Work out the finished part from the listing and answer in its coordinate system (mm). Give positions to 0.01 mm unless a question says otherwise; leave off trailing zeros. Loops run counter-clockwise (first coordinate to the right, second up) from the corner with the lowest first, then second, coordinate; pieces in that order, holes last. Notation, with made-up numbers: (45.25, -24) - (90.25, -24) arc R9 ccw to (90.25, -18) - close; hole circle Ø10 at (63, 83). An arc over 180 degrees is marked (long way). One line per item, written item: value.
from build123d import *

# Parameters (mm, degrees)
PAD_DEPTH    = 0.046
SKETCH002_W  = 1.924742
SKETCH002_H  = 2.351108
PAD001_DEPTH = 0.05
SKETCH003_W  = 0.414509
SKETCH003_H  = 1.190033
PAD002_DEPTH = 0.05


with BuildPart() as part:
    # Sketch → Pad (new body)
    with BuildSketch(Plane.XY):
        Polygon((36.346094, 51.80915), (36.392998, 51.701576), (36.392998, 51.109999), (37.742998, 51.109999), (37.742998, 51.259997), (38.392999, 51.259997), (38.392999, 49.31), (35.458194, 49.31), (35.4573, 49.310176), (35.427625, 49.310087), (35.398525, 49.315875), (34.512999, 49.315875), (34.395946, 49.292591), (34.296711, 49.226287), (34.230407, 49.127052), (34.207122, 49.009999), (34.207122, 45.461999), (34.230407, 45.344946), (34.296711, 45.245711), (34.386002, 45.186051), (34.386002, 44.708), (34.642999, 44.708), (34.642999, 44.322444), (34.615783, 44.295228), (34.565999, 44.175042), (34.565999, 44.044954), (34.615783, 43.924769), (34.642999, 43.897553), (34.642999, 38.31), (34.992186, 38.31), (34.992186, 36.056903), (36.893, 36.056903), (36.893, 35.478903), (36.871742, 35.372032), (36.871742, 33.780103), (36.890262, 33.687001), (36.860833, 33.559999), (33.906066, 33.559999), (33.906066, 35.790099), (33.069934, 35.790099), (33.069934, 34.437018), (33.064958, 34.412001), (33.064958, 33.673212), (32.951745, 33.559999), (31.092999, 33.559999), (31.092999, 50.109999), (28.362245, 50.109999), (28.362245, 53.56), (31.439899, 53.56), (31.439899, 51.809147), align=None)
    extrude(amount=PAD_DEPTH)

    # Sketch002 (on Face52 of Pad) → Pad001 (join)
    with BuildSketch(Plane.XY.offset(0.046)):
        with Locations((29.62901, 51.992506)):
            Rectangle(SKETCH002_W, SKETCH002_H)
    extrude(amount=PAD001_DEPTH)

    # Sketch003 (on Face5 of Pad001) → Pad002 (join)
    with BuildSketch(Plane.XY.offset(0.046)):
        with Locations((34.881022, 34.35564)):
            Rectangle(SKETCH003_W, SKETCH003_H)
    extrude(amount=PAD002_DEPTH)


solid = part.part
1. A flat-ended cylindrical pin translates along its axis: pin 1 Ø1.5 at (x, y) = (32.5, 42.5) entering from +Z. Find the tip coordinate at first contact, or state that the pin passes through.
Output:
pin 1: stops at z = 0.05
2. Section C-C (y = 46.75) is taken. Write down the section's boundary in (x, z), and give its area (3 significant figures).
Output:
outline: (31.09, 0) - (34.21, 0) - (34.21, 0.05) - (31.09, 0.05) - close
area: 0.143 mm²
3. Section A-A (x = 29.75) is taken. Write down the section's boundary in (y, z).
Output:
outline: (50.11, 0) - (53.56, 0) - (53.56, 0.05) - (53.17, 0.05) - (53.17, 0.1) - (50.82, 0.1) - (50.82, 0.05) - (50.11, 0.05) - close
4. Section B-B (y = 40) is taken. Write down the section's boundary in (x, z).
Output:
outline: (31.09, 0) - (34.64, 0) - (34.64, 0.05) - (31.09, 0.05) - close
